Autodesk Inventor part; units mm, degrees
ref_plane "YZ Plane" through (0, 0, 0) normal (1, 0, 0) x (0, 1, 0)
ref_plane "XZ Plane" through (0, 0, 0) normal (0, 1, 0) x (-1, 0, 0)
ref_plane "XY Plane" through (0, 0, 0) normal (0, 0, 1) x (1, 0, 0)
sketch "Sketch1" plane through (0, 0, 0) normal (0, 0, 1) x (1, 0, 0)
  line L0 (0, 0) -> (-90.17, 0)
  line L1 (-90.17, 0) -> (-90.17, 31.75)
  line L2 (-90.17, 31.75) -> (0, 31.75)
  line L3 (0, 31.75) -> (0, 0)
  dimension "d0" = 90.17
  dimension "d1" = 31.75
extrude "Extrusion1" add sketch "Sketch1" against normal blind 25.4
sketch "Sketch2" plane through (-90.17, 31.75, 0) normal (0, 1, 0) x (1, 0, 0)
  line L0 (0, 0) -> (90.17, 0)
  line L1 (90.17, 0) -> (90.17, 25.4)
  line L2 (0, 25.4) -> (90.17, 25.4)
  line L3 (0, 0) -> (0, 25.4)
  line L4 (90.17, 0) -> (52.07, 0)
  line L5 (52.07, 0) -> (52.07, 25.4)
  line L6 (52.07, 25.4) -> (90.17, 25.4)
  line L7 (90.17, 25.4) -> (90.17, 0)
  line L8 (0, 0) -> (0, 25.4)
  line L9 (0, 0) -> (38.1, 0)
  line L10 (38.1, 0) -> (38.1, 25.4)
  line L11 (38.1, 25.4) -> (0, 25.4)
  line L12 (0, 25.4) -> (0, 0)
  line L13 (38.1, 6.223) -> (52.07, 6.223)
  line L14 (52.07, 6.223) -> (52.07, 19.177)
  line L15 (52.07, 19.177) -> (38.1, 19.177)
  line L16 (38.1, 19.177) -> (38.1, 6.223)
  circle A0 centre (45.085, 12.7) radius 6.477
  line L17 (35.433, 6.223) -> (54.737, 6.223)
  line L18 (54.737, 6.223) -> (54.737, 19.177)
  line L19 (54.737, 19.177) -> (35.433, 19.177)
  line L20 (35.433, 19.177) -> (35.433, 6.223)
  dimension "d4" = 38.1
  dimension "d5" = 38.1
  dimension "d6" = 6.223
  dimension "d7" = 6.223
  dimension "d8" = 6.477
  dimension "d10" = 6.985
  dimension "d11" = 6.985
  dimension "d12" = 12.954
  dimension "d15" = 3.175
  dimension "d16" = 3.175
extrude "Extrusion2" cut sketch "Sketch2" against normal blind 76.2 contours A0
sketch "Sketch3" plane through (-90.17, 31.75, 0) normal (0, 1, 0) x (1, 0, 0)
  circle A0 centre (45.085, 12.7) radius 6.477
  line L0 (35.433, 6.223) -> (54.737, 6.223)
  line L1 (54.737, 6.223) -> (54.737, 19.177)
  line L2 (54.737, 19.177) -> (35.433, 19.177)
  line L3 (35.433, 19.177) -> (35.433, 6.223)
  dimension "d17" = 0
  dimension "d18" = 0
  dimension "d19" = 3.175
  dimension "d20" = 3.175
extrude "Extrusion3" cut sketch "Sketch3" against normal blind 76.2 contours A0 L2 L1 L0 | A0 L0 L3 L2
properties part number "Lidar Holder 1"
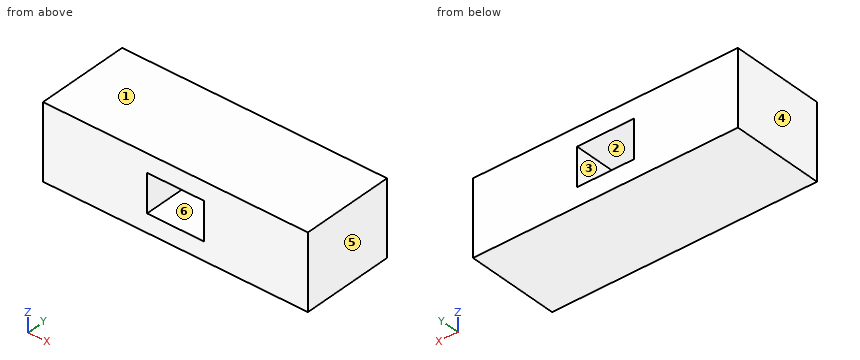
CAD build for the part. Positions are in the model's coordinates, mm. Face numbers are marked on the shaded views. A direction names the side the tool comes from. Round coordinates to 2 decimals unless told otherwise and drop trailing zeros. Loops run counter-clockwise (first coordinate to the right, second up) from the corner with the lowest first, then second, coordinate; pieces in that order, holes last. Notation, with made-up numbers: M -35,-14.75 L -28,-14.75 A35 ccw -28,20.25 Z; hole C -22.5,-5 d7. An arc over 180 degrees is marked long. One line per question, with ' | ' between items. Start each with the question number.
Item 1: Cut at C-C, the plane y = 13. Write the cut outline in (x, z), plus the area to 3 significant figures.
Item 2: Which spindle directions (+Z, -Z, +X, -X, +Y, -Y) get a long thin tool onto all of the face, cutting with end or side? Do the marked faces 5 and 6. Say none if no direction does.
Item 3: Cut at A-A, the plane x = -38. Write the cut outline in (y, z), plus the area to 3 significant figures.
Item 4: Two-plate mould, pull along Z, no slides. Class the marked faces 1, 2, 3 and 4: pulls with the +Z half, pulls with the -Z half, needs draft (parallel to the pull), parting line crosses it, or undercut.
Item 5: Wall check: line 1 (Z direction, x = -45, y = 7); line 2 (X direction, y = 13.5, z = -16). Give the ranges that are in metal, low to high.
Item 6: Cut at B-B, the plane z = -8. Write the cut outline in (x, y).
Responses:
1) outline: M -90.17,-25.4 L 0,-25.4 L 0,0 L -90.17,0 Z; hole M -54.74,-19.18 L -35.43,-19.18 L -35.43,-6.22 L -54.74,-6.22 Z | area: 2,040 mm²
2) face 5: +Z, -Z, +X, +Y, -Y | face 6: +Y, -Y
3) outline: M 0,-25.4 L 31.75,-25.4 L 31.75,-19.18 L 0,-19.18 Z; M 0,-6.22 L 31.75,-6.22 L 31.75,0 L 0,0 Z | area: 395 mm²
4) face 1: pulls with the +Z half | face 2: undercut | face 3: undercut | face 4: needs draft
5) line 1: z = -25.4 to -19.18, -6.22 to 0 | line 2: x = -90.17 to -54.74, -35.43 to 0
6) outline: M -90.17,0 L -54.74,0 L -54.74,31.75 L -90.17,31.75 Z; M -35.43,0 L 0,0 L 0,31.75 L -35.43,31.75 Z
